Work out the finished part from the listing and answer in its coordinate system (mm). A direction names the side the tool comes from. Round coordinates to 2 decimals unless told otherwise and drop trailing zeros. Write each loop counter-clockwise with the first axis right and the second up, starting at its lowest first coordinate (ties: lowest second). Pieces come first, ordered by that corner, then holes. Notation, with made-up numbers: (55.25, -22.75) - (82.25, -22.75) arc R11 ccw to (82.25, -6.75) - close; hole circle Ø6 at (18.5, -22.75). An arc over 180 degrees is marked (long way). Answer as a JSON object with one key per item and string values.
```python
from build123d import *

# Parameters (mm, degrees)
SKETCH1_R           = 3
SKETCH1_R_2         = 1.5
BOSS_EXTRUDE1_DEPTH = 3
SKETCH2_R           = 4.440231585
SKETCH2_R_2         = 1.5
BOSS_EXTRUDE2_DEPTH = 2
FILLET1_R           = 3


with BuildPart() as part:
    # Sketch1 → Boss-Extrude1 (new body)
    with BuildSketch(Plane.XY):
        with BuildLine():
            Line((-33.316424849, 111.282839546), (-70.905727769, 115.89291218))
            ThreePointArc((-70.905727769, 115.89291218), (-79.948137164, 106.850502785), (-70.905727769, 97.808093391))
            Line((-70.905727769, 97.808093391), (-33.676430248, 102.388731808))
            Line((-33.676430248, 102.388731808), (-32.956569458, 102.477302429))
            ThreePointArc((-32.956569458, 102.477302429), (-29.398198623, 107.032843823), (-33.316424849, 111.282839546))
        make_face()
        with Locations((-70.905727769, 106.850502785)):
            Circle(SKETCH1_R, mode=Mode.SUBTRACT)
        with BuildLine():
            ThreePointArc((-45.817442834, 108.585056612), (-44.082889007, 106.850502785), (-45.817442834, 105.115948958))
            Line((-45.817442834, 105.115948958), (-58.948305776, 105.115948958))
            ThreePointArc((-58.948305776, 105.115948958), (-60.682859603, 106.850502785), (-58.948305776, 108.585056612))
            Line((-58.948305776, 108.585056613), (-45.817442834, 108.585056613))
        make_face(mode=Mode.SUBTRACT)
        with Locations((-33.860020841, 106.850502785)):
            Circle(SKETCH1_R_2, mode=Mode.SUBTRACT)
    extrude(amount=BOSS_EXTRUDE1_DEPTH)

    # Sketch2 → Boss-Extrude2 (add)
    with BuildSketch(Plane.XY.offset(3)):
        with Locations((-70.905727769, 106.850502785)):
            Circle(SKETCH2_R)
        with Locations((-70.905727769, 106.850502785)):
            Circle(SKETCH2_R_2, mode=Mode.SUBTRACT)
    extrude(amount=BOSS_EXTRUDE2_DEPTH)

    # Fillet1
    # the kernel refuses this fillet: 3 mm, written as the material it adds along each edge
    with BuildSketch(Plane(origin=(-70.905727769, 106.850502785, 3), x_dir=(1, 0, 0), z_dir=(0, -1, 0))) as fillet1_piece_1:
        with BuildLine():
            CenterArc((7.26865871, 3), FILLET1_R, 199.471220634, 70.528779366)
            Line((4.440231585, 2), (4.383663043, 1.98))
            ThreePointArc((4.383663043, 1.98), (4.380231585, 1), (4.380231585, 0))
            Line((4.380231585, 0), (4.440231585, -0.06))
            Line((4.440231585, -0.06), (7.26865871, -0.06))
            Line((7.26865871, -0.06), (7.26865871, 0))
        make_face()
    revolve(axis=Axis((-70.905727769, 106.850502785, 3), (0, 0, 1)))


solid = part.part
```
Item 1: A cutting plane is placed at C-C (z = 4.05). Write down the section's boundary in (x, y).
Results found:
{"outline": "circle Ø9.98 at (-70.91, 106.85); hole circle Ø3 at (-70.91, 106.85)"}
Item 2: A cutting plane is placed at A-A (z = 1.15). Write down the section's boundary in (x, y).
Results found:
{"outline": "(-70.91, 97.81) - (-32.96, 102.48) arc R4.47 ccw to (-33.32, 111.28) - (-70.91, 115.89) arc R9.04 ccw to start; hole circle Ø6 at (-70.91, 106.85); hole (-58.95, 105.12) - (-45.82, 105.12) arc R1.73 ccw to (-45.82, 108.59) - (-58.95, 108.59) arc R1.73 ccw to start; hole circle Ø3 at (-33.86, 106.85)"}
Item 3: A cutting plane is placed at B-B (y = 106.25). Give the number of separate pieces and of enclosed holes in the cut face, and give its area (3 significant figures).
Results found:
{"separate pieces": "4", "enclosed holes": "0", "area": "91.6 mm²"}
Item 4: Consider line 1 along Z through (x, y) = (-44, 109.5); line 2 along Y through (x, z) = (-69.5, 2.55); line 3 along Y through (x, z) = (-48.5, 2.85) (3 decimals). Determine where each line is inside the solid, lowest interval first.
Results found:
{"line 1": "0 to 3", "line 2": "97.98 to 104.2, 109.5 to 115.72", "line 3": "100.565 to 105.116, 108.585 to 113.145"}
Item 5: A cutting plane is placed at D-D (y = 114.75). Write down the section's boundary in (x, z), and give its area (3 significant figures).
Results found:
{"outline": "(-75.31, 0) - (-61.59, 0) - (-61.59, 3) - (-75.31, 3) - close", "area": "41.2 mm²"}
Item 6: Determine the mould class of faces 4 (the cylindrical face through (-33.17, 105.52, 1.48)), 5 (the flat face through (-51.848, 113.556, 1.479)), 6 (the flat face through (-71, 105, 5)) for opening direction Y: pulls with the +Y half, pulls with the -Y half, needs draft (parallel to the pull), parting line crosses it, or undercut.
Results found:
{"face 4": "undercut", "face 5": "pulls with the +Y half", "face 6": "needs draft"}
Item 7: Each of these flat-tipped pins is pushed along its axis until it touches: P1, Ø0.9, axis at x = -55, z = 2, coming from the -Y side; P2, Ø5, axis at x = -70.91, y = 106.85, coming from the -Z side; P3, Ø5.5, axis at x = -56.5, y = 105.5, coming from the +Z side; P4, Ø2.5, axis at x = -33.86, y = 106.85, coming from the -Z side. Where does it stop, or does it pass through?
Results found:
{"P1": "y = 99.71", "P2": "z = 3", "P3": "z = 3", "P4": "through"}
Item 8: For faces 1 (the cylindrical face through (-73.29, 105.03, 1.48)), 2 (the flat face through (-52, 105.116, 1)), 3 (the cylindrical face through (-79.946, 107.049, 1.479)), determine the directions among +Z, -Z, +X, -X, +Y, -Y from which every point of the face is accessible in a straight line to the end or side of a thin tool.
Results found:
{"face 1": "-Z", "face 2": "+Z, -Z", "face 3": "+Z, -Z, -X"}
